from build123d import *

# Parameters (mm, degrees)
BOSS_EXTRUDE1_START      = -23110
BOSS_EXTRUDE1_DEPTH      = 5
BOSS_EXTRUDE1_DEPTH_BACK = 100
SKETCH3_W                = 150.118051911
SKETCH3_H                = 92.714651823
BOSS_EXTRUDE2_DEPTH      = 20
SKETCH4_R                = 10
BOSS_EXTRUDE3_DEPTH      = 50


with BuildPart() as part:
    # Sketch2 → Boss-Extrude1 (new body, two sides)
    with BuildSketch(Plane(origin=(0, 0, 0), x_dir=(0, 0, -1), z_dir=(1, 0, 0)).offset(BOSS_EXTRUDE1_START)) as boss_extrude1_sk:
        Polygon((-40429.816686048, 2996.894248022), (-40415.674550424, 3011.036383646), (-40415.674550424, 2982.752112399), align=None)
        Polygon((-40072.930236915, 2640.00779889), (-40415.674550424, 2982.752112399), (-40415.674550424, 3011.036383646), (-40072.930236915, 2668.292070137), align=None)
        Polygon((-40058.788101291, 2654.149934513), (-40072.930236915, 2640.00779889), (-40072.930236915, 2668.292070137), align=None)
    extrude(amount=BOSS_EXTRUDE1_DEPTH)
    extrude(boss_extrude1_sk.sketch, amount=-BOSS_EXTRUDE1_DEPTH_BACK)

    # Sketch3 → Boss-Extrude2 (add)
    with BuildSketch(Plane(origin=(0, -18716.461219013, 18716.461219015), x_dir=(1, 0, 0), z_dir=(0, -0.707106781, 0.707106781))):
        with Locations((-23029.940974045, 30660.964460197)):
            Rectangle(SKETCH3_W, SKETCH3_H)
        with Locations((-23029.940974045, 30248.965455429)):
            Rectangle(SKETCH3_W, SKETCH3_H)
    extrude(amount=-BOSS_EXTRUDE2_DEPTH)

    # Sketch4 → Boss-Extrude3 (add)
    with BuildSketch(Plane(origin=(0, -18702.319083389, 18702.319083389), x_dir=(1, 0, 0), z_dir=(0, 0.707106781, -0.707106781))):
        with Locations((-23146.230449039, -30340.794679614)):
            Circle(SKETCH4_R)
        with Locations((-23146.230449039, -30520.794679614)):
            Circle(SKETCH4_R)
    extrude(amount=BOSS_EXTRUDE3_DEPTH)


solid = part.part
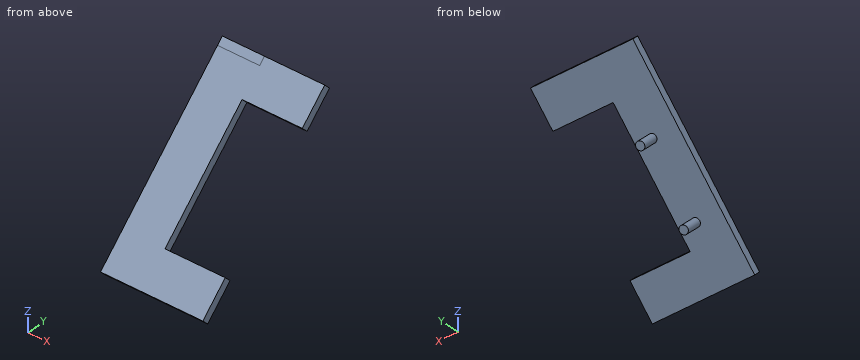
Read the model definition and answer for the solid it produces. Units are mm, in the model's axes. Round coordinates to 2 decimals unless told otherwise and drop trailing zeros. Order: outer loops, then holes, each group sorted by start corner. A loop starts at its lowest first (then second) coordinate and runs counter-clockwise, first axis right, second up.
1) The part is cut by section C-C on y = 2825.5. Write down the section's boundary in (x, z).
2) The part is cut by section A-A on x = -23043. Write down the section's boundary in (y, z).
3) Straight lines are drawn through the part: L1, parallel to Y at x = -23154.5, z = 40144 (3 decimals); L2, parallel to X at y = 2822, z = 40231; L3, parallel to Y at x = -23105, z = 40374.5. For each, find the intervals that lie inside material, in ascending order.
4) Flat-ended cylindrical pins translate along their axes: pin 1 (10 mm diameter, centred on x = -23016, z = 40115, fed in from -Y); pin 2 (3 mm diameter, centred on x = -23145.5, z = 40294, fed in from +Y); pin 3 (5 mm diameter, centred on y = 2890, z = 40257, fed in from +X). Find the tip coordinate at first contact, or state that the pin passes through.
5) The part is cut by section D-D on z = 40381.5. Write down the section's boundary in (x, y), plus the area to 3 significant figures.
6) The part is cut by section B-B on x = -23149.5. Write down the section's boundary in (y, z), plus the area to 3 significant figures.
Resolved:
1. outline: (-23210, 40230.14) - (-23105, 40230.14) - (-23105, 40258.42) - (-23210, 40258.42) - close
2. outline: (2640.01, 40072.93) - (2654.15, 40058.79) - (2719.71, 40124.35) - (2705.57, 40138.49) - close; (2931.34, 40364.26) - (2945.48, 40350.12) - (3011.04, 40415.67) - (2996.89, 40429.82) - close
3. L1: y = 2711.078 to 2739.362, 2756.412 to 2772.315
3. L2: x = -23210 to -23105
3. L3: y = 2941.58 to 2969.86
4. pin 1: stops at y = 2677.08
4. pin 2: stops at y = 2890.86
4. pin 3: stops at x = -23141.4
5. outline: (-23210, 2948.58) - (-22954.88, 2948.58) - (-22954.88, 2976.86) - (-23210, 2976.86) - close
5. area: 7,220 mm2
6. outline: (2640.01, 40072.93) - (2654.15, 40058.79) - (2745.18, 40149.82) - (2780.54, 40114.46) - (2793.9, 40127.83) - (2758.55, 40163.18) - (2872.46, 40277.1) - (2907.81, 40241.74) - (2921.18, 40255.11) - (2885.82, 40290.46) - (3011.04, 40415.67) - (2996.89, 40429.82) - close
6. area: 12,000 mm2
